Part print with two shaded views. Sizes in mm from the minimum x, y, z corner. Coordinates: 2 decimals unless noted, no trailing zeros. Write each loop counter-clockwise with the first axis right and the second up, starting at its lowest first coordinate (ties: lowest second). Pieces come first, ordered by that corner, then holes. Notation, with made-up numbers: (-15, 79.25) - (14, 79.25) arc R31 cw to (14, 106.25) - close; hole circle Ø7 at (52.25, 7.25). An arc over 180 degrees is marked (long way). One line per question, with ' | ' between items. Start each with the question number.
1. Band-saw the part on C-C, the plane y = 34. Write the cut outline in (x, z), then the cut area to 3 significant figures.
2. Band-saw the part on A-A, the plane z = 13.25. Write the cut outline in (x, y), then the cut area to 3 significant figures.
3. Flat gauge pins, fed straight in: P1, Ø2, axis at x = 788.5, z = 10, coming from the +Y side; P2, Ø3, axis at x = 766.5, z = 5, coming from the +Y side; P3, Ø8, axis at x = 264, z = 13.5, coming from the +Y side. Where does each tip first touch, or does it go through?
4. Probe line 1 (Y direction, x = 620, z = 10.5); line 2 (Y direction, x = 464.5, z = 11.5). List the from-to ranges inside material, lowest first.
5. Band-saw the part on B-B, the plane x = 370.5. Write the cut outline in (y, z), then the cut area to 3 significant figures.
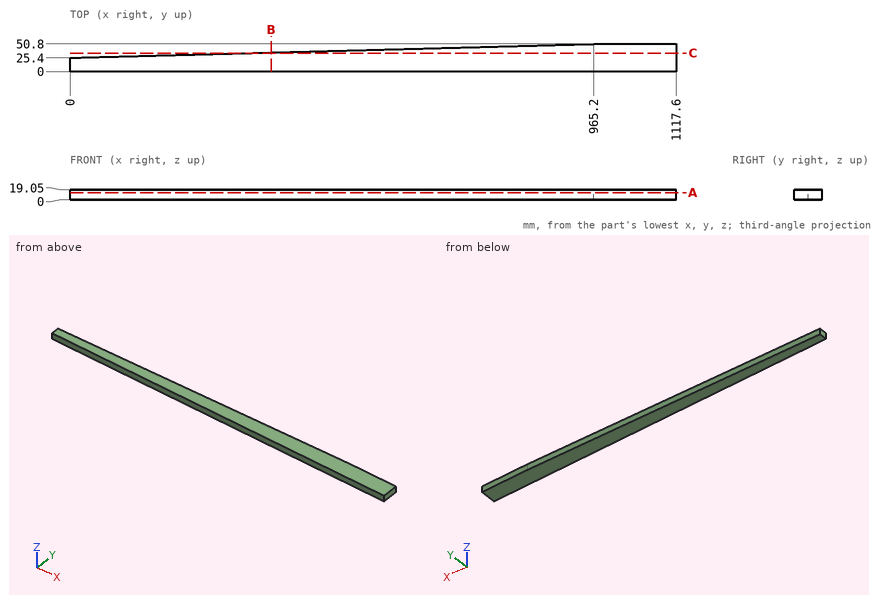
Filled in:
1) outline: (326.8, 0) - (1117.6, 0) - (1117.6, 19.05) - (326.8, 19.05) - close | area: 15,100 mm²
2) outline: (0, 0) - (1117.6, 0) - (1117.6, 50.8) - (965.2, 50.8) - (0, 25.4) - close | area: 44,500 mm²
3) P1: stops at y = 46.18 | P2: stops at y = 45.61 | P3: stops at y = 32.45
4) line 1: y = 0 to 41.72 | line 2: y = 0 to 37.62
5) outline: (0, 0) - (35.15, 0) - (35.15, 19.05) - (0, 19.05) - close | area: 670 mm²
